Design review of the part shown in the three views and the two pictorial views. Dimensions are in mm from the part's minimum x, y and z. Round coordinates to 2 decimals unless told otherwise and drop trailing zeros. Order: outer loops, then holes, each group sorted by start corner. A loop starts at its lowest first (then second) coordinate and runs counter-clockwise, first axis right, second up. Notation, with made-up numbers: (87, 67.5) - (99, 67.5) arc R28 cw to (99, 99.5) - close; hole circle Ø11 at (38.25, 81). An arc over 180 degrees is marked (long way). Use CSV: the item, a comma, the result in double quotes.
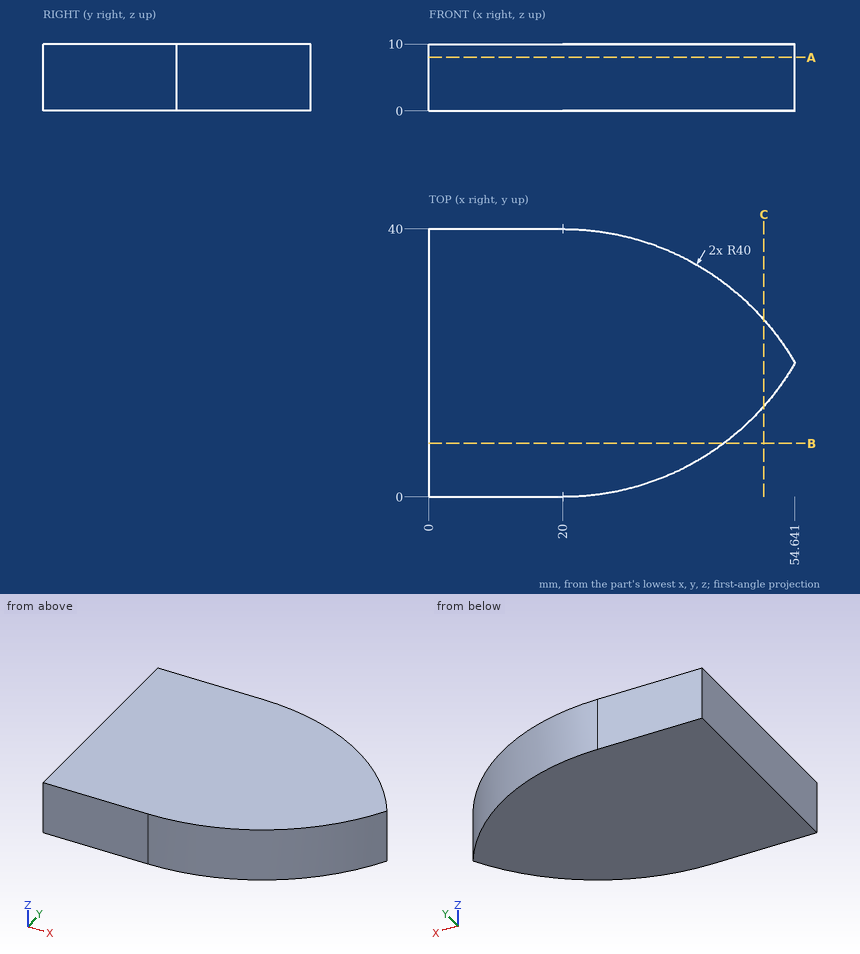
1) To check wall thickness, follow L1, parallel to X at y = 17, z = 1.25; L2, parallel to X at y = 22.5, z = 3.5; L3, parallel to Y at x = 38.5, z = 4.25. State the ranges of each line that lie inside material, in increasing order. Write a range as from..to.
Data:
L1,"x = 0..52.73"
L2,"x = 0..53.07"
L3,"y = 4.54..35.46"
2) Insertion check: pin 1 Ø4 at (y, z) = (17, 5) entering from +X; pin 2 Ø5 at (y, z) = (10, 7.5) entering from +X; pin 3 Ø2 at (x, z) = (34, 8.5) entering from +Y. Each pin has a flat end and moves straight along its axis. Give the tip position at first contact, or say it passes through.
Data:
pin 1,"stops at x = 54.04"
pin 2,"stops at x = 49.05"
pin 3,"stops at y = 37.83"
3) We need section B-B (y = 8). Give the boundary of the cut face in (x, z).
Data:
outline,"(0, 0) - (44, 0) - (44, 10) - (0, 10) - close"
4) We need section A-A (z = 8). Give the boundary of the cut face in (x, y).
Data:
outline,"(0, 0) - (20, 0) arc R40 ccw to (54.64, 20) arc R40 ccw to (20, 40) - (0, 40) - close"
5) We need section C-C (x = 50). Give the boundary of the cut face in (y, z), then the cut area to 3 significant figures.
Data:
outline,"(13.54, 0) - (26.46, 0) - (26.46, 10) - (13.54, 10) - close"
area,"129 mm2"
